from build123d import *

# Parameters (mm, degrees)
SKETCH1_W                = 20
SKETCH1_H                = 42
SKETCH1_W_2              = 42
BOSS_EXTRUDE1_DEPTH      = 6
SKETCH2_R                = 11.25
CUT_EXTRUDE1_DEPTH       = 3
CUT_EXTRUDE2_DEPTH       = 47.454278597
CUT_EXTRUDE2_DEPTH_BACK  = 47.454278597
SKETCH3_R                = 1.75
SKETCH3_R_2              = 6
CUT_EXTRUDE3_START       = -3
SKETCH4_R                = 3
SKETCH4_R_2              = 1.75
CUT_EXTRUDE3_DEPTH       = 3
SKETCH5_W                = 4.5
SKETCH5_H                = 42
BOSS_EXTRUDE2_DEPTH      = 3
CHAMFER1_SIZE            = 3
CUT_EXTRUDE4_DEPTH       = 47.936126811
CUT_EXTRUDE4_DEPTH_BACK  = 47.936126811
SKETCH6_R                = 2.75
SKETCH7_W                = 9.456435582
SKETCH7_H                = 20
SKETCH7_R                = 2.75
CUT_EXTRUDE5_DEPTH       = 47.454278597
BOSS_EXTRUDE4_DEPTH      = 3
BOSS_EXTRUDE4_DEPTH_BACK = 6
SKETCH8_W                = 20
SKETCH8_H                = 42
SKETCH8_R                = 7
CHAMFER2_SIZE            = 4
SKETCH9_R                = 50
CUT_EXTRUDE7_DEPTH       = 1.5
CUT_EXTRUDE8_START       = -1.5
SKETCH10_R               = 3
CUT_EXTRUDE8_DEPTH       = 1.5
CUT_EXTRUDE9_START       = -3
SKETCH11_R               = 7
CUT_EXTRUDE9_DEPTH       = 3


with BuildPart() as part:
    # Sketch1 → Boss-Extrude1 (new body)
    with BuildSketch(Plane.XY):
        with Locations((31, 0)):
            Rectangle(SKETCH1_W, SKETCH1_H)
        Rectangle(SKETCH1_W_2, SKETCH1_H)
    extrude(amount=BOSS_EXTRUDE1_DEPTH)

    # Sketch2 → Cut-Extrude1 (cut)
    with BuildSketch(Plane.XY):
        Circle(SKETCH2_R)
    extrude(amount=CUT_EXTRUDE1_DEPTH, mode=Mode.SUBTRACT)

    # Sketch3 → Cut-Extrude2 (cut, two sides: drawn at the far end of the back side and taken through both)
    with BuildSketch(Plane.XY.offset(-CUT_EXTRUDE2_DEPTH_BACK)):
        with Locations((-15.499780644, 15.499780644)):
            Circle(SKETCH3_R)
        Circle(SKETCH3_R_2)
        with Locations((15.499780644, 15.499780644)):
            Circle(SKETCH3_R)
        with Locations((15.499780644, -15.499780644)):
            Circle(SKETCH3_R)
        with Locations((-15.499780644, -15.499780644)):
            Circle(SKETCH3_R)
    extrude(amount=CUT_EXTRUDE2_DEPTH + CUT_EXTRUDE2_DEPTH_BACK, mode=Mode.SUBTRACT)

    # Sketch4 → Cut-Extrude3 (cut)
    # profile 1 of 4: a face of its own
    with BuildSketch(Plane.XY.offset(6).offset(CUT_EXTRUDE3_START)):
        with Locations((-15.499780644, -15.499780644)):
            Circle(SKETCH4_R)
        with Locations((-15.499780644, -15.499780644)):
            Circle(SKETCH4_R_2, mode=Mode.SUBTRACT)
    # profile 2 of 4: a face of its own
    with BuildSketch(Plane.XY.offset(6).offset(CUT_EXTRUDE3_START)):
        with Locations((-15.499780644, 15.499780644)):
            Circle(SKETCH4_R)
        with Locations((-15.499780644, 15.499780644)):
            Circle(SKETCH4_R_2, mode=Mode.SUBTRACT)
    # profile 3 of 4: a face of its own
    with BuildSketch(Plane.XY.offset(6).offset(CUT_EXTRUDE3_START)):
        with Locations((15.499780644, 15.499780644)):
            Circle(SKETCH4_R)
        with Locations((15.499780644, 15.499780644)):
            Circle(SKETCH4_R_2, mode=Mode.SUBTRACT)
    # profile 4 of 4: a face of its own
    with BuildSketch(Plane.XY.offset(6).offset(CUT_EXTRUDE3_START)):
        with Locations((15.499780644, -15.499780644)):
            Circle(SKETCH4_R)
        with Locations((15.499780644, -15.499780644)):
            Circle(SKETCH4_R_2, mode=Mode.SUBTRACT)
    extrude(amount=CUT_EXTRUDE3_DEPTH, mode=Mode.SUBTRACT)

    # Sketch5 → Boss-Extrude2 (add)
    with BuildSketch(Plane.XY.offset(6)):
        with Locations((31, 0)):
            Rectangle(SKETCH5_W, SKETCH5_H)
    extrude(amount=BOSS_EXTRUDE2_DEPTH)

    # Chamfer1
    chamfer1_edges = [part.edges().sort_by_distance(p)[0] for p in [
        (-21, -21, 3),
        (-21, 21, 3),
    ]]
    chamfer(chamfer1_edges, length=CHAMFER1_SIZE)

    # Sketch6 → Cut-Extrude4 (cut, two sides: drawn at the far end of the back side and taken through both)
    with BuildSketch(Plane(origin=(0, 0, 0), x_dir=(-1, 0, 0), z_dir=(0, 0, -1)).offset(-CUT_EXTRUDE4_DEPTH_BACK)):
        with Locations(Location((-31, 0, 0), (0, 0, 324.903198772))):
            Circle(SKETCH6_R)
    extrude(amount=CUT_EXTRUDE4_DEPTH + CUT_EXTRUDE4_DEPTH_BACK, mode=Mode.SUBTRACT)

    # Sketch7 → Cut-Extrude5 (cut, through all)
    with BuildSketch(Plane.XY.offset(6)):
        with Locations((31, 0)):
            Rectangle(SKETCH7_W, SKETCH7_H)
        with Locations((31, 0)):
            Circle(SKETCH7_R, mode=Mode.SUBTRACT)
    extrude(amount=CUT_EXTRUDE5_DEPTH, mode=Mode.SUBTRACT)

    # Sketch8 → Boss-Extrude4 (add, two sides: drawn at the far end of the back side and taken through both)
    # profile 1 of 2: a face of its own
    with BuildSketch(Plane(origin=(0, 0, 0), x_dir=(-1, 0, 0), z_dir=(0, 0, -1)).offset(-BOSS_EXTRUDE4_DEPTH_BACK)):
        Polygon((18, -21), (-21, -21), (-41, -21), (-41, -24), (24, -24), (24, 24), (-41, 24), (-41, 21), (-21, 21), (18, 21), (21, 18), (21, -18), align=None)
    # profile 2 of 2: a face of its own
    with BuildSketch(Plane(origin=(0, 0, 0), x_dir=(-1, 0, 0), z_dir=(0, 0, -1)).offset(-BOSS_EXTRUDE4_DEPTH_BACK)):
        with Locations((-31, 0)):
            Rectangle(SKETCH8_W, SKETCH8_H)
        with Locations((-31, 0)):
            Circle(SKETCH8_R, mode=Mode.SUBTRACT)
    extrude(amount=BOSS_EXTRUDE4_DEPTH + BOSS_EXTRUDE4_DEPTH_BACK)

    # Chamfer2
    chamfer2_edges = [part.edges().sort_by_distance(p)[0] for p in [
        (-24, 24, 1.5),
        (-24, -24, 1.5),
    ]]
    chamfer(chamfer2_edges, length=CHAMFER2_SIZE)

    # Sketch9 → Cut-Extrude7 (cut)
    with BuildSketch(Plane.XY.offset(6)):
        with Locations((-40, 0)):
            Circle(SKETCH9_R)
    extrude(amount=-CUT_EXTRUDE7_DEPTH, mode=Mode.SUBTRACT)

    # Sketch10 → Cut-Extrude8 (cut)
    with BuildSketch(Plane.XY.offset(3).offset(CUT_EXTRUDE8_START)):
        with Locations((-15.499780644, 15.499780644)):
            Circle(SKETCH10_R)
        with Locations((-15.499780644, -15.499780644)):
            Circle(SKETCH10_R)
    extrude(amount=CUT_EXTRUDE8_DEPTH, mode=Mode.SUBTRACT)

    # Sketch11 → Cut-Extrude9 (cut)
    with BuildSketch(Plane(origin=(0, 0, 0), x_dir=(-1, 0, 0), z_dir=(0, 0, -1)).offset(CUT_EXTRUDE9_START)):
        with Locations((-31, 0)):
            Circle(SKETCH11_R)
    extrude(amount=CUT_EXTRUDE9_DEPTH, mode=Mode.SUBTRACT)


solid = part.part
Design review of the part built by this model. Coordinates are the model's own, in mm. A direction names the side the tool comes from. Coordinates: 2 decimals unless noted, no trailing zeros. Loops run counter-clockwise (first coordinate to the right, second up) from the corner with the lowest first, then second, coordinate; pieces in that order, holes last. Notation, with made-up numbers: (32.5, -19) - (80.5, -19) arc R17 cw to (80.5, -6) - close; hole circle Ø2 at (86, -16.75). An arc over 180 degrees is marked (long way). Use CSV: the item, a comma, the result in double quotes. Start each with the question number.
1. To check wall thickness, follow probe 1 along Y at (x, z) = (31, 4.5); probe 2 along X at (y, z) = (1, 1.75); probe 3 along X at (y, z) = (14.5, 1.25). State the ranges of each line that lie inside material, in increasing order.
2. Add section A-A on z = -2. Give the boundary of the cut face in (x, y), plus the area to 3 significant figures.
3. Add section B-B on z = 6.75. Give the boundary of the cut face in (x, y).
4. For faces 1 (the cylindrical face through (10, 0, 5)), 2 (the flat face through (-20, -19, -1)), 3 (the flat face through (31, -21, 7)), 4 (the flat face through (-14, -17, 1.5)), list the 3-axis set-ups (+Z, -Z, +X, -X, +Y, -Y) from which the entire face can be reached by the end or side of a thin tool; tool diameter is ignored.
5. Mouldability with a two-part tool opening along Y and no side actions: class faces 5 (the flat face through (10, 24, 2)), 6 (the cylindrical face through (5.19, -9.98, 1.48)), 7 (the cylindrical face through (-17.9, 13.7, 3)), 8 (the flat face through (23, 6, -3)) as released by +Y, released by -Y, zero draft, split by the parting line, or undercut.
6. Clearance check with flat-ended pins moving along their axes: pin 1 (2 mm diameter, centred on x = 5, y = 15.5, fed in from +Z); pin 2 (2.5 mm diameter, centred on x = 31, z = 7.5, fed in from -Y); pin 3 (4 mm diameter, centred on x = 26.5, y = 9.5, fed in from +Z). State where each tip first meets the part, or that it passes through.
7. Add section C-C on y = 0. Give the boundary of the cut face in (x, z).
8. Add section D-D on x = 31. Give the boundary of the cut face in (y, z).
Resolved:
1,probe 1,"-24 to -2.75, 2.75 to 24"
1,probe 2,"-24 to -11.21, 11.21 to 24.07, 37.93 to 41"
1,probe 3,"-24 to -16.94, -14.06 to 14.06, 16.94 to 41"
2,outline,"(-24, -20) - (-20, -24) - (41, -24) - (41, 24) - (-20, 24) - (-24, 20) - close; hole (-21, -18) - (-18, -21) - (21, -21) - (21, 21) - (-18, 21) - (-21, 18) - close; hole circle Ø14 at (31, 0)"
2,area,"1,200 mm2"
3,outline,"(28.75, -21) - (33.25, -21) - (33.25, -10) - (28.75, -10) - close; (28.75, 10) - (33.25, 10) - (33.25, 21) - (28.75, 21) - close"
4,face 1,"+Z, -X"
4,face 2,"-Z"
4,face 3,"+Z, +X, -X, -Y"
4,face 4,"+Z"
5,face 5,"released by +Y"
5,face 6,"undercut"
5,face 7,"undercut"
5,face 8,"zero draft"
6,pin 1,"z = 4.5"
6,pin 2,"y = -21"
6,pin 3,"z = 6"
7,outline,"(-24, -3) - (-21, -3) - (-21, 0) - (-11.25, 0) - (-11.25, 3) - (-6, 3) - (-6, 4.5) - (-24, 4.5) - close; (6, 3) - (11.25, 3) - (11.25, 0) - (21, 0) - (21, -3) - (24, -3) - (24, 3) - (28.25, 3) - (28.25, 6) - (10, 6) - (10, 4.5) - (6, 4.5) - close; (33.75, 3) - (38, 3) - (38, -3) - (41, -3) - (41, 6) - (33.75, 6) - close"
8,outline,"(-24, -3) - (-7, -3) - (-7, 3) - (-2.75, 3) - (-2.75, 6) - (-10, 6) - (-10, 9) - (-21, 9) - (-21, 6) - (-24, 6) - close; (2.75, 3) - (7, 3) - (7, -3) - (24, -3) - (24, 6) - (21, 6) - (21, 9) - (10, 9) - (10, 6) - (2.75, 6) - close"
